CAD build for the part. Positions are in the model's coordinates, mm. Give positions to 0.01 mm unless a question says otherwise; leave off trailing zeros. Write each loop counter-clockwise with the first axis right and the second up, starting at its lowest first coordinate (ties: lowest second). Pieces come first, ordered by that corner, then holes. Notation, with made-up numbers: (30, 21) - (62, 21) arc R15 cw to (62, 30) - close; hole circle Ø2 at (72, 80). An arc over 180 degrees is marked (long way). Answer as a JSON object with one key per item and string values.
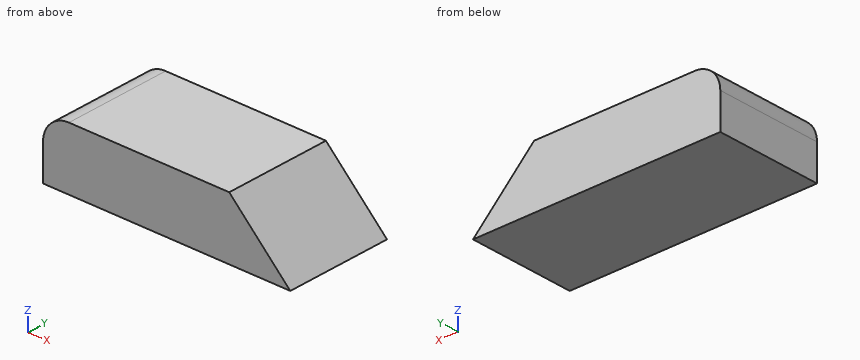
from build123d import *

# Parameters (mm, degrees)
F0_W        = 599.3404984474
F0_H        = 229.6551764011
F1_DEPTH    = 131
F2_R        = 55.5269119346
F3_T1_DEPTH = 1258.3283715875


# Not quite as in the source:
# - a fillet or chamfer that OpenCascade refuses, or shapes differently, is made with other operations: its cross-section is extruded or revolved along the edge and cut away or added


with BuildPart() as f1:
    # F0 (on Top) → F1 (new body)
    with BuildSketch(Plane.XY):
        with Locations((-30.9103131294, -57.0044666529)):
            Rectangle(F0_W, F0_H)
    extrude(amount=F1_DEPTH)

    # F2
    f2_edges = [f1.edges().sort_by_distance(p)[0] for p in [
        (-330.580562, -57.004467, 131),
    ]]
    fillet(f2_edges, radius=F2_R)

    # F3: chamfer of 200 on 1 edges, made by hand

    # F3_s2 → F3_t1 (cut)
    with BuildSketch(Plane.XZ.offset(-572.1597191409)):
        Polygon((68.7599360943, 131), (268.7599360943, -69), (268.7599360943, 131), align=None)
    extrude(amount=F3_T1_DEPTH, mode=Mode.SUBTRACT)


solid = f1.part
(1) Flat gauge pin, fed straight in: P1, Ø3, axis at x = 125, y = -59, coming from the +Z side. Where does the tip first touch, or does it go through?
Answer key:
{"P1": "stops at z = 76.26"}
(2) Probe L1, parallel to X at y = 44, z = 24.5; L2, parallel to Z at x = 128, y = -32; L3, parallel to X at y = -149.5, z = 115. List the from-to ranges inside material, lowest first. Write a range as [from, to].
Answer key:
{"L1": "x = [-330.58, 175.26]", "L2": "z = [0, 71.76]", "L3": "x = [-314.05, 84.76]"}
(3) Saw through at C-C, the plane x = 94. Give the cut face in (y, z), and give its area (3 significant figures).
Answer key:
{"outline": "(-171.83, 0) - (57.82, 0) - (57.82, 105.76) - (-171.83, 105.76) - close", "area": "24,300 mm²"}
(4) Saw through at A-A, the plane y = -1. Give the cut face in (x, z).
Answer key:
{"outline": "(-330.58, 0) - (199.76, 0) - (68.76, 131) - (-275.05, 131) arc R55.53 ccw to (-330.58, 75.47) - close"}
(5) Saw through at B-B, the plane z = 13.5. Give the cut face in (x, y).
Answer key:
{"outline": "(-330.58, -171.83) - (186.26, -171.83) - (186.26, 57.82) - (-330.58, 57.82) - close"}
